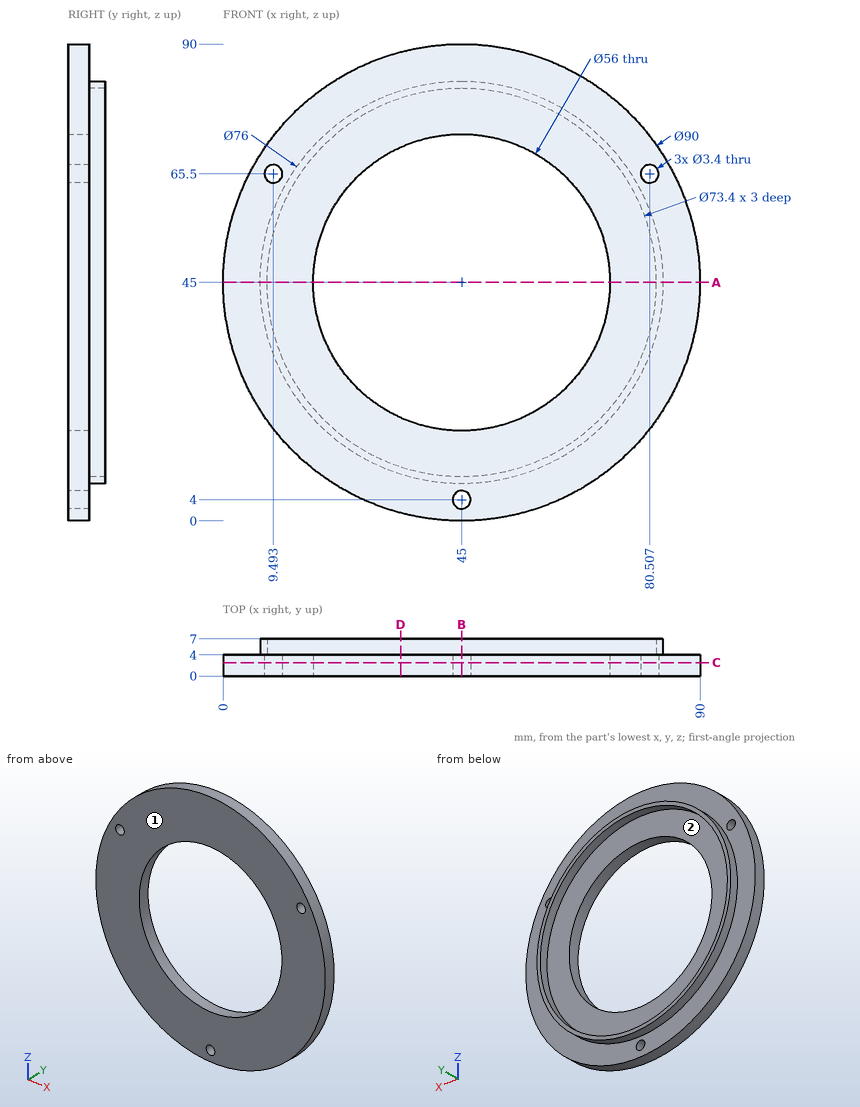
For this review, use the dimensioned drawing (mm, ordinates from the lowest corner) and the shaded views. Round coordinates to 2 decimals unless told otherwise and drop trailing zeros. Write each loop counter-clockwise with the first axis right and the second up, starting at its lowest first coordinate (ties: lowest second). Pieces come first, ordered by that corner, then holes. Notation, with made-up numbers: (-9, -23.5) - (50, -23.5) arc R23 ccw to (50, -0.5) - close; hole circle Ø6 at (61.25, -16.5). An arc over 180 degrees is marked (long way). One line per item, written item: value. Start each with the question number.
1. Consider section A-A on z = 45. Write out the cut boundary in (x, y).
2. Consider section D-D on x = 33.5. Write out the cut boundary in (y, z), and give its area (3 significant figures).
3. Clearance check with flat-ended pins moving along their axes: P1, Ø4.5, axis at x = 80.51, z = 65.5, coming from the +Y side; P2, Ø1, axis at y = 1, z = 60, coming from the +X side; P3, Ø4, axis at x = 54.5, y = 2.5, coming from the -Z side. State where each tip first meets the part, or that it passes through.
4. Consider section B-B on x = 45. Write out the cut boundary in (y, z), and give its area (3 significant figures).
5. To check wall thickness, follow L1, parallel to X at y = 3.2, z = 45; L2, parallel to X at y = 3.2, z = 65.5; L3, parallel to Y at x = 85, z = 41. State the ranges of each line that lie inside material, in increasing order. Write a range as from..to.
6. The part is to be moulded in two halves that separate along X. For the marked faces 1 and 2, say which applies: released by +X, released by -X, zero draft, split by the parting line, or undercut.
7. Consider section C-C on y = 2.5. Write out the cut boundary in (x, z), and give its area (3 significant figures).
Checks:
1. outline: (0, 0) - (17, 0) - (17, 4) - (8.3, 4) - (8.3, 7) - (7, 7) - (7, 4) - (0, 4) - close; (73, 0) - (90, 0) - (90, 4) - (83, 4) - (83, 7) - (81.7, 7) - (81.7, 4) - (73, 4) - close
2. outline: (0, 1.49) - (4, 1.49) - (4, 8.78) - (7, 8.78) - (7, 10.15) - (4, 10.15) - (4, 19.47) - (0, 19.47) - close; (0, 70.53) - (4, 70.53) - (4, 79.85) - (7, 79.85) - (7, 81.22) - (4, 81.22) - (4, 88.51) - (0, 88.51) - close
2. area: 152 mm^2
3. P1: stops at y = 4
3. P2: stops at x = 87.6
3. P3: stops at z = 0.63
4. outline: (0, 0) - (4, 0) - (4, 2.3) - (0, 2.3) - close; (0, 5.7) - (4, 5.7) - (4, 7) - (7, 7) - (7, 8.3) - (4, 8.3) - (4, 17) - (0, 17) - close; (0, 73) - (4, 73) - (4, 81.7) - (7, 81.7) - (7, 83) - (4, 83) - (4, 90) - (0, 90) - close
4. area: 130 mm^2
5. L1: x = 0..17, 73..90
5. L2: x = 4.94..7.79, 11.19..25.93, 64.07..78.81, 82.21..85.06
5. L3: y = 0..4
6. face 1: zero draft
6. face 2: undercut
7. outline: circle Ø90 at (45, 45); hole circle Ø3.4 at (9.49, 65.5); hole circle Ø56 at (45, 45); hole circle Ø3.4 at (45, 4); hole circle Ø3.4 at (80.51, 65.5)
7. area: 3,870 mm^2
